Geometry: final body of the model. Coordinates: model frame, mm. Face numbers are marked on the shaded views. A direction names the side the tool comes from. Give positions to 0.01 mm unless a question says otherwise; leave off trailing zeros. Order: outer loops, then holes, each group sorted by start corner. A loop starts at its lowest first (then second) coordinate and runs counter-clockwise, first axis right, second up. Notation, with made-up numbers: (54, -25.75) - (74, -25.75) arc R18 ccw to (74, -0.75) - close; hole circle Ø11 at (74.25, 26.25). An arc over 180 degrees is marked (long way). Put each result on its own line as item: value. Start each with the question number.
1. Mould query, pull axis Z, two halves, no side actions, for the marked faces 1, 2, 3 and 4. Classes: pulls with the +Z half, pulls with the -Z half, needs draft (parallel to the pull), parting line crosses it, or undercut.
2. Section B-B on z = 25.5. Return the cut outline in (x, y) (3 decimals).
3. First-contact query: P1, Ø6, axis at x = 62.5, z = -33.5, coming from the +Y side; P2, Ø6.5, axis at x = 83.5, y = -8.5, coming from the -Z side (3 decimals); P3, Ø7.5, axis at x = 90, z = 10.5, coming from the -Y side. Flat tips, straight axial feed; report the tip coordinate or a pass-through.
4. Section D-D on x = 43. Return the cut outline in (y, z) (3 decimals), plus the area to 3 significant figures.
5. Ray query, line 1 along X through (y, z) = (-6, 32) (3 decimals); line 2 along X through (y, z) = (8, -0.5) (3 decimals); line 3 along X through (y, z) = (-42.5, -51.5) (3 decimals). Return the intervals inside material, ascending. Write a range as from..to.
6. Set-up query: the marked faces 5, 6 and 7. Return all of +Z, -Z, +X, -X, +Y, -Y with unobstructed straight access to the full face (end or side cutting, diameter ignored); none if empty.
7. Section C-C on y = -6.35. Return the cut outline in (x, z) (3 decimals).
8. Section A-A on y = 101.6. Return the cut outline in (x, z) (3 decimals), plus the area to 3 significant figures.
from build123d import *

# Parameters (mm, degrees)
SKETCH1_W                   = 196.85
SKETCH1_H                   = 82.55
BOSS_EXTRUDE1_DEPTH         = 95.25
SKETCH3_W                   = 146.05
SKETCH3_H                   = 76.2
CUT_EXTRUDE1_DEPTH          = 144.051280141
SKETCH4_W                   = 25.4
SKETCH4_H                   = 53.975
BOSS_EXTRUDE2_DEPTH         = 6.35
SKETCH5_W                   = 25.4
SKETCH5_H                   = 12.7
BOSS_EXTRUDE3_DEPTH         = 25.4
SKETCH6_W                   = 26.67
SKETCH6_H                   = 2.54
CUT_EXTRUDE2_DEPTH          = 229.622047548
F_1_4_0_25_DIAMETER_HOLE1_D = 6.35
SKETCH16_W                  = 196.85
SKETCH16_H                  = 6.35
CUT_EXTRUDE3_DEPTH          = 191.790819682
BOSS_EXTRUDE4_START         = -6.35
SKETCH11_W                  = 25.4
SKETCH11_H                  = 12.7
BOSS_EXTRUDE4_DEPTH         = 6.35
F_8_CLEARANCE_HOLE1_D       = 4.4958
F_8_CLEARANCE_HOLE1_DEPTH   = 12.7
SKETCH14_W                  = 146.05
SKETCH14_H                  = 41.275
BOSS_EXTRUDE5_DEPTH         = 6.35


with BuildPart() as part:
    # Sketch1 → Boss-Extrude1 (new body)
    with BuildSketch(Plane(origin=(0, 0, 0), x_dir=(1, 0, 0), z_dir=(0, 1, 0))):
        Rectangle(SKETCH1_W, SKETCH1_H)
    extrude(amount=BOSS_EXTRUDE1_DEPTH)

    # Sketch3 → Cut-Extrude1 (cut, through all)
    with BuildSketch(Plane(origin=(0, 95.25, 0), x_dir=(1, 0, 0), z_dir=(0, 1, 0))):
        with Locations((0, -3.175)):
            Rectangle(SKETCH3_W, SKETCH3_H)
    extrude(amount=-CUT_EXTRUDE1_DEPTH, mode=Mode.SUBTRACT)

    # Sketch4 → Boss-Extrude2 (add)
    with BuildSketch(Plane(origin=(0, 0, -41.275), x_dir=(-1, 0, 0), z_dir=(0, 0, -1))):
        with Locations((-85.725, -26.9875)):
            Rectangle(SKETCH4_W, SKETCH4_H)
    boss_extrude2 = extrude(amount=-BOSS_EXTRUDE2_DEPTH)

    # Sketch5 → Boss-Extrude3 (add)
    with BuildSketch(Plane(origin=(0, 0, -41.275), x_dir=(-1, 0, 0), z_dir=(0, 0, -1))):
        with Locations((-85.725, -47.625)):
            Rectangle(SKETCH5_W, SKETCH5_H)
    boss_extrude3 = extrude(amount=BOSS_EXTRUDE3_DEPTH)

    # Sketch6 → Cut-Extrude2 (cut, through all)
    with BuildSketch(Plane(origin=(98.425, 0, 0), x_dir=(0, 0, -1), z_dir=(1, 0, 0))):
        with Locations((50.8, -52.705)):
            Rectangle(SKETCH6_W, SKETCH6_H)
    cut_extrude2 = extrude(amount=-CUT_EXTRUDE2_DEPTH, mode=Mode.SUBTRACT)

    # 1/4 (0.25) Diameter Hole1 (through all)
    with Locations(Plane(origin=(0, -41.275, 0), x_dir=(1, 0, 0), z_dir=(0, 1, 0))):
        with Locations((85.725, 53.975)):
            f_1_4_0_25_diameter_hole1 = Hole(F_1_4_0_25_DIAMETER_HOLE1_D / 2)

    # Sketch16 → Cut-Extrude3 (cut, through all)
    with BuildSketch(Plane(origin=(0, 95.25, 0), x_dir=(1, 0, 0), z_dir=(0, 1, 0))):
        with Locations((0, -38.1)):
            Rectangle(SKETCH16_W, SKETCH16_H)
    extrude(amount=-CUT_EXTRUDE3_DEPTH, mode=Mode.SUBTRACT)

    # Sketch11 → Boss-Extrude4 (add)
    with BuildSketch(Plane.XY.offset(41.275).offset(BOSS_EXTRUDE4_START)):
        with Locations((85.725, 101.6)):
            Rectangle(SKETCH11_W, SKETCH11_H)
        with Locations((85.725, -6.35)):
            Rectangle(SKETCH11_W, SKETCH11_H)
    boss_extrude4 = extrude(amount=-BOSS_EXTRUDE4_DEPTH)

    # #8 Clearance Hole1
    with Locations(Plane.XY.offset(41.275)):
        with Locations((85.725, 101.6), (85.725, -6.35)):
            f_8_clearance_hole1 = Hole(F_8_CLEARANCE_HOLE1_D / 2, depth=F_8_CLEARANCE_HOLE1_DEPTH)

    # Mirror1: Boss-Extrude2, Boss-Extrude3, Cut-Extrude2, 1/4 (0.25) Diameter Hole1, Boss-Extrude4, #8 Clearance Hole1 across plane
    add(boss_extrude2.mirror(Plane(origin=(0, 0, 0), x_dir=(0, 0, 1), z_dir=(1, 0, 0))))
    add(boss_extrude3.mirror(Plane(origin=(0, 0, 0), x_dir=(0, 0, 1), z_dir=(1, 0, 0))))
    add(cut_extrude2.mirror(Plane(origin=(0, 0, 0), x_dir=(0, 0, 1), z_dir=(1, 0, 0))), mode=Mode.SUBTRACT)
    add(f_1_4_0_25_diameter_hole1.mirror(Plane(origin=(0, 0, 0), x_dir=(0, 0, 1), z_dir=(1, 0, 0))), mode=Mode.SUBTRACT)
    add(boss_extrude4.mirror(Plane(origin=(0, 0, 0), x_dir=(0, 0, 1), z_dir=(1, 0, 0))))
    add(f_8_clearance_hole1.mirror(Plane(origin=(0, 0, 0), x_dir=(0, 0, 1), z_dir=(1, 0, 0))), mode=Mode.SUBTRACT)

    # Sketch14 → Boss-Extrude5 (add)
    with BuildSketch(Plane(origin=(0, 0, -41.275), x_dir=(-1, 0, 0), z_dir=(0, 0, -1))):
        with Locations((0, -20.6375)):
            Rectangle(SKETCH14_W, SKETCH14_H)
    extrude(amount=-BOSS_EXTRUDE5_DEPTH)


solid = part.part
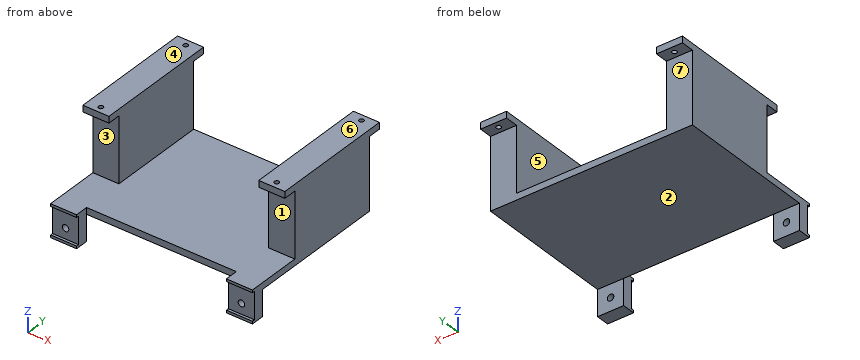
Resolved:
1. face 1: undercut
1. face 2: pulls with the -Z half
1. face 3: undercut
1. face 4: pulls with the +Z half
2. outline: (-98.425, 0) - (-73.025, 0) - (-73.025, 95.25) - (-98.425, 95.25) - close; (73.025, 0) - (98.425, 0) - (98.425, 95.25) - (73.025, 95.25) - close
3. P1: y = 95.25
3. P2: z = -41.275
3. P3: y = 0
4. outline: (-41.275, -41.275) - (95.25, -41.275) - (95.25, -34.925) - (-41.275, -34.925) - close
4. area: 867 mm^2
5. line 1: -98.425..-87.945, -83.505..-73.025, 73.025..83.505, 87.945..98.425
5. line 2: -98.425..-73.025, 73.025..98.425
5. line 3: -98.425..-87.714, -83.736..-73.025, 73.025..83.736, 87.714..98.425
6. face 5: +Z, +Y, -Y
6. face 6: +Z, +X, -X, +Y, -Y
6. face 7: -Z, +X, -X, +Y
7. outline: (-98.425, -41.275) - (98.425, -41.275) - (98.425, -34.925) - (-98.425, -34.925) - close; (-98.425, 28.575) - (-87.973, 28.575) - (-87.973, 34.925) - (-98.425, 34.925) - close; (-83.477, 28.575) - (-73.025, 28.575) - (-73.025, 34.925) - (-83.477, 34.925) - close; (73.025, 28.575) - (83.477, 28.575) - (83.477, 34.925) - (73.025, 34.925) - close; (87.973, 28.575) - (98.425, 28.575) - (98.425, 34.925) - (87.973, 34.925) - close
8. outline: (-98.425, 28.575) - (-87.973, 28.575) - (-87.973, 34.925) - (-98.425, 34.925) - close; (-83.477, 28.575) - (-73.025, 28.575) - (-73.025, 34.925) - (-83.477, 34.925) - close; (73.025, 28.575) - (83.477, 28.575) - (83.477, 34.925) - (73.025, 34.925) - close; (87.973, 28.575) - (98.425, 28.575) - (98.425, 34.925) - (87.973, 34.925) - close
8. area: 265 mm^2
